from build123d import *

# Parameters (mm, degrees)
SKETCH1_W           = 203.2
SKETCH1_H           = 50.8
BOSS_EXTRUDE1_DEPTH = 2.54


with BuildPart() as part:
    # Sketch1 → Boss-Extrude1 (new body)
    with BuildSketch(Plane.XY.offset(111.506)):
        with Locations((27.742628903, 3.491347131)):
            Rectangle(SKETCH1_W, SKETCH1_H)
        with BuildLine():
            Line((-52.164996369, 5.396347131), (107.650254176, 5.396347131))
            ThreePointArc((107.650254176, 5.396347131), (109.555254176, 3.491347131), (107.650254176, 1.586347131))
            Line((107.650254176, 1.586347131), (-52.164996369, 1.586347131))
            ThreePointArc((-52.164996369, 1.586347131), (-54.069996369, 3.491347131), (-52.164996369, 5.396347131))
        make_face(mode=Mode.SUBTRACT)
    extrude(amount=-BOSS_EXTRUDE1_DEPTH)


solid = part.part
The listing builds one solid part. Answer for the finished solid, in the listing's coordinates (mm). Give positions to 0.01 mm unless a question says otherwise; leave off trailing zeros. Loops run counter-clockwise (first coordinate to the right, second up) from the corner with the lowest first, then second, coordinate; pieces in that order, holes last. Notation, with made-up numbers: (27, 49) - (66, 49) arc R21 cw to (66, 63) - close; hole circle Ø6 at (33.25, 3). An arc over 180 degrees is marked (long way). Answer as a JSON object with one key per item and string values.
1. A cutting plane is placed at A-A (x = 26.5). Write down the section's boundary in (y, z), then the cut area to 3 significant figures.
Determined:
{"outline": "(-21.91, 108.97) - (1.59, 108.97) - (1.59, 111.51) - (-21.91, 111.51) - close; (5.4, 108.97) - (28.89, 108.97) - (28.89, 111.51) - (5.4, 111.51) - close", "area": "119 mm²"}
2. Find the intervals of material crossed by L1, parallel to Y at x = 5, z = 110.7; L2, parallel to X at y = 2, z = 110.95; L3, parallel to X at y = 4, z = 109.9, in increasing order. Write a range as [from, to].
Determined:
{"L1": "[-21.91, 1.59], [5.4, 28.89]", "L2": "[-73.86, -53.35], [108.84, 129.34]", "L3": "[-73.86, -54], [109.49, 129.34]"}
3. A cutting plane is placed at B-B (z = 111). Write down the section's boundary in (x, y) (3 decimals).
Determined:
{"outline": "(-73.857, -21.909) - (129.343, -21.909) - (129.343, 28.891) - (-73.857, 28.891) - close; hole (-52.165, 1.586) - (107.65, 1.586) arc R1.905 ccw to (107.65, 5.396) - (-52.165, 5.396) arc R1.905 ccw to start"}
